```python
from build123d import *

# Parameters (mm, degrees)
SKETCH018_R          = 7.5
PAD_DEPTH            = 2
CHAMFER_SIZE         = 0.75
CHAMFER001_SIZE      = 0.75
SKETCH019_R          = 8.401279
POCKET015_DEPTH      = 2.001
POCKET015_DEPTH_BACK = 0.001
SKETCH020_R          = 5
POCKET016_DEPTH      = 0.001
POCKET016_DEPTH_BACK = 2.001


with BuildPart() as part:
    # Sketch018 → Pad (new body)
    with BuildSketch(Plane.XY):
        Circle(SKETCH018_R)
    extrude(amount=PAD_DEPTH)

    # Chamfer
    chamfer_edges = [part.edges().sort_by_distance(p)[0] for p in [
        (-7.5, 0, 2),
    ]]
    chamfer(chamfer_edges, length=CHAMFER_SIZE)

    # Chamfer001
    chamfer001_edges = [part.edges().sort_by_distance(p)[0] for p in [
        (-7.5, 0, 0),
    ]]
    chamfer(chamfer001_edges, length=CHAMFER001_SIZE)

    # Sketch019 (on Face3 of Pad) → Pocket015 (cut, two sides)
    with BuildSketch(Plane.XY.offset(2)) as pocket015_sk:
        Circle(SKETCH019_R)
        Polygon((0, 7.332348), (-6.35, 3.666174), (-6.35, -3.666174), (0, -7.332348), (6.35, -3.666174), (6.35, 3.666174), align=None, mode=Mode.SUBTRACT)
    extrude(amount=-POCKET015_DEPTH, mode=Mode.SUBTRACT)
    extrude(pocket015_sk.sketch, amount=POCKET015_DEPTH_BACK, mode=Mode.SUBTRACT)

    # Sketch020 → Pocket016 (cut, two sides)
    with BuildSketch(Plane.XY) as pocket016_sk:
        Circle(SKETCH020_R)
    extrude(amount=-POCKET016_DEPTH, mode=Mode.SUBTRACT)
    extrude(pocket016_sk.sketch, amount=POCKET016_DEPTH_BACK, mode=Mode.SUBTRACT)


solid = part.part
```
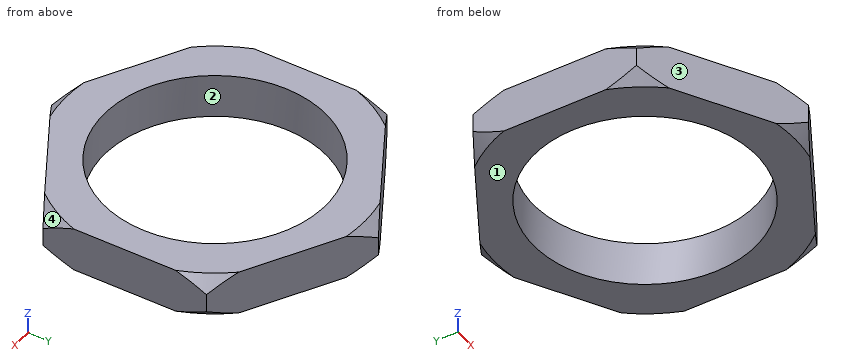
Verification items for the finished model (mm, model axes). Face numbers are marked on the shaded views. Round coordinates to 2 decimals unless told otherwise and drop trailing zeros. Write each loop counter-clockwise with the first axis right and the second up, starting at its lowest first coordinate (ties: lowest second). Pieces come first, ordered by that corner, then holes.
1. Draft check along X on the marked faces 1, 2, 3 and 4. Enter one of: +X half, -X half, draft (parallel to the pull), parting line (faces both ways), or undercut.
2. Section check B-B on x = -3.5. Enter the section's corners in (y, z), plus the area to 3 significant figures.
3. Section check A-A on y = 0. Enter the section's corners in (x, z).
4. Scan lines: L1, parallel to X at y = 0, z = 0.45; L2, parallel to Y at x = 1.75, z = 1.65; L3, parallel to Y at x = -4, z = 1.35. Record each from-to range of solid material in increasing order.
5. Section check C-C on z = 1.8. Enter the section's corners in (x, y), plus the area to 3 significant figures.
Answer:
1. face 1: draft
1. face 2: undercut
1. face 3: -X half
1. face 4: +X half
2. outline: (-5.31, 0) - (-3.57, 0) - (-3.57, 2) - (-5.31, 2) - close; (3.57, 0) - (5.31, 0) - (5.31, 2) - (3.57, 2) - close
2. area: 6.96 mm2
3. outline: (-6.35, 0) - (-5, 0) - (-5, 2) - (-6.35, 2) - close; (5, 0) - (6.35, 0) - (6.35, 2) - (5, 2) - close
4. L1: x = -6.35 to -5, 5 to 6.35
4. L2: y = -6.32 to -4.68, 4.68 to 6.32
4. L3: y = -5.02 to -3, 3 to 5.02
5. outline: (-6.35, -2.82) arc R6.95 ccw to (-5.62, -4.09) - (-0.73, -6.91) arc R6.95 ccw to (0.73, -6.91) - (5.62, -4.09) arc R6.95 ccw to (6.35, -2.82) - (6.35, 2.82) arc R6.95 ccw to (5.62, 4.09) - (0.73, 6.91) arc R6.95 ccw to (-0.73, 6.91) - (-5.62, 4.09) arc R6.95 ccw to (-6.35, 2.82) - close; hole circle Ø10 at (0, 0)
5. area: 59.5 mm2
